```python
from build123d import *

# Parameters (mm, degrees)
SKETCH1_R                  = 45
SKETCH1_R_2                = 5
BOSS_EXTRUDE1_DEPTH        = 8
F_4_3_4_3_DIAMETER_HOLE1_D = 4.3
SKETCH6_R                  = 30.1
SKETCH6_R_2                = 19.9
CUT_EXTRUDE2_DEPTH         = 1.5
SKETCH8_R                  = 24
SKETCH8_R_2                = 12.5
CUT_EXTRUDE3_DEPTH         = 3
SKETCH9_R                  = 24
SKETCH9_R_2                = 14.5
CUT_EXTRUDE4_DEPTH         = 0.6
SKETCH10_R                 = 12.5
SKETCH10_R_2               = 2.15
BOSS_EXTRUDE2_DEPTH        = 14.5
CHAMFER1_SIZE              = 1
FILLET1_R                  = 1


with BuildPart() as part:
    # Sketch1 → Boss-Extrude1 (new body)
    with BuildSketch(Plane(origin=(0, 0, 0), x_dir=(1, 0, 0), z_dir=(0, 1, 0))):
        with Locations(Location((0, 0, 0), (0, 0, 270))):
            Circle(SKETCH1_R)
        with Locations(Location((0, 36.5, 0), (0, 0, 270))):
            Circle(SKETCH1_R_2, mode=Mode.SUBTRACT)
        with Locations(Location((34.713562845, 11.279120295, 0), (0, 0, 270))):
            Circle(SKETCH1_R_2, mode=Mode.SUBTRACT)
        with Locations(Location((21.454161709, -29.529120295, 0), (0, 0, 270))):
            Circle(SKETCH1_R_2, mode=Mode.SUBTRACT)
        with Locations(Location((-21.454161709, -29.529120295, 0), (0, 0, 270))):
            Circle(SKETCH1_R_2, mode=Mode.SUBTRACT)
        with Locations(Location((-34.713562845, 11.279120295, 0), (0, 0, 270))):
            Circle(SKETCH1_R_2, mode=Mode.SUBTRACT)
    extrude(amount=BOSS_EXTRUDE1_DEPTH)

    # Ø4.3 (4.3) Diameter Hole1 (through all)
    with Locations(Plane(origin=(0, 8, 0), x_dir=(1, 0, 0), z_dir=(0, 1, 0))):
        with Locations((-7.60845213, -2.472135955), (-4.702282018, 6.472135955), (4.702282018, 6.472135955), (7.60845213, -2.472135955), (0, -8)):
            Hole(F_4_3_4_3_DIAMETER_HOLE1_D / 2)

    # Sketch6 → Cut-Extrude2 (cut)
    with BuildSketch(Plane.XZ):
        with Locations(Location((0, 0, 0), (0, 0, 270))):
            Circle(SKETCH6_R)
        with Locations(Location((0, 0, 0), (0, 0, 270))):
            Circle(SKETCH6_R_2, mode=Mode.SUBTRACT)
    extrude(amount=-CUT_EXTRUDE2_DEPTH, mode=Mode.SUBTRACT)

    # Sketch8 → Cut-Extrude3 (cut)
    with BuildSketch(Plane(origin=(0, 8, 0), x_dir=(1, 0, 0), z_dir=(0, 1, 0))):
        with Locations(Location((0, 0, 0), (0, 0, 270))):
            Circle(SKETCH8_R)
        with Locations(Location((0, 0, 0), (0, 0, 270))):
            Circle(SKETCH8_R_2, mode=Mode.SUBTRACT)
    extrude(amount=-CUT_EXTRUDE3_DEPTH, mode=Mode.SUBTRACT)

    # Sketch9 → Cut-Extrude4 (cut)
    with BuildSketch(Plane(origin=(0, 5, 0), x_dir=(1, 0, 0), z_dir=(0, 1, 0))):
        with Locations(Location((0, 0, 0), (0, 0, 270))):
            Circle(SKETCH9_R)
        with Locations(Location((0, 0, 0), (0, 0, 270))):
            Circle(SKETCH9_R_2, mode=Mode.SUBTRACT)
    extrude(amount=-CUT_EXTRUDE4_DEPTH, mode=Mode.SUBTRACT)

    # Sketch10 → Boss-Extrude2 (add)
    with BuildSketch(Plane.XZ.offset(-8)):
        with Locations(Location((0, 0, 0), (0, 0, 90))):
            Circle(SKETCH10_R)
        with Locations(Location((7.60845213, 2.472135955, 0), (0, 0, 90))):
            Circle(SKETCH10_R_2, mode=Mode.SUBTRACT)
        with Locations(Location((4.702282018, -6.472135955, 0), (0, 0, 90))):
            Circle(SKETCH10_R_2, mode=Mode.SUBTRACT)
        with Locations(Location((-4.702282018, -6.472135955, 0), (0, 0, 90))):
            Circle(SKETCH10_R_2, mode=Mode.SUBTRACT)
        with Locations(Location((-7.60845213, 2.472135955, 0), (0, 0, 90))):
            Circle(SKETCH10_R_2, mode=Mode.SUBTRACT)
        with Locations(Location((0, 8, 0), (0, 0, 90))):
            Circle(SKETCH10_R_2, mode=Mode.SUBTRACT)
    extrude(amount=-BOSS_EXTRUDE2_DEPTH)

    # Chamfer1
    chamfer1_edges = [part.edges().sort_by_distance(p)[0] for p in [
        (0, 22.5, -12.5),
    ]]
    chamfer(chamfer1_edges, length=CHAMFER1_SIZE)

    # Sketch11 → Cut-Revolve1 (revolve, cut)
    with BuildSketch(Plane.XY, mode=Mode.PRIVATE) as cut_revolve1_sk:
        Polygon((12.5, 5), (12.5, 7), (10.5, 5), align=None)
    revolve(cut_revolve1_sk.sketch.rotate(Axis((0, 1.5, 0), (0, -1, 0)), 90), axis=Axis((0, 1.5, 0), (0, -1, 0)), mode=Mode.SUBTRACT)

    # Fillet1
    fillet1_edges = [part.edges().sort_by_distance(p)[0] for p in [
        (0, 5, -10.5),
    ]]
    fillet(fillet1_edges, radius=FILLET1_R)


solid = part.part
```
Check sheet for the modelled part. Datum: model origin and axes. Units: mm. A direction names the side the tool comes from. Give positions to 0.01 mm unless a question says otherwise; leave off trailing zeros. Order: outer loops, then holes, each group sorted by start corner. A loop starts at its lowest first (then second) coordinate and runs counter-clockwise, first axis right, second up. Notation, with made-up numbers: (-33, -10.75) -> (-27, -10.75) arc R20 ccw to (-27, 23.25) -> close; hole circle Ø3 at (28, 19). An arc over 180 degrees is marked (long way). Use CSV: the item, a comma, the result in double quotes. Start each with the question number.
1) Material ranges on line 1 (X direction, y = 7.5, z = -4); line 2 (Z direction, x = -12, y = 4.5); line 3 (X direction, y = 2, z = 34), recorded low to high. Write a range as from..to.
2) Sectioned sample at B-B, the plane x = -38. Record the boundary of the cut face in (y, z).
3) Set-up check for faces 1 (the face through (-29.384, 0.74, 6.525)), 2 (the face through (9, 5, 10)), 3 (the face through (-0.8, 11.092, 9.996)): record each of +Z, -Z, +X, -X, +Y, -Y from which the full face is reachable in a straight line by a thin tool's end or side.
4) Sectioned sample at A-A, the plane z = -36.5. Record the boundary of the cut face in (x, y).
5) Go/stop test with flat-tipped pins: P1, Ø16, axis at x = -21.45, z = 29.53, coming from the +Y side; P2, Ø6, axis at x = 15, z = -18.5, coming from the -Y side; P3, Ø8, axis at x = 3, y = 11, coming from the +Z side. Record where each tip stops, or that it passes through.
6) Sectioned sample at C-C, the plane y = 17.25. Record the boundary of the cut face in (x, z), plus the area to 3 significant figures.
7) Sectioned sample at D-D, the plane z = -26. Record the boundary of the cut face in (x, y).
Recorded:
1,line 1,"-44.82..-23.66, -11.84..11.84, 23.66..44.82"
1,line 2,"-43.37..-20.78, -8.14..8.14, 20.78..43.37"
1,line 3,"-29.48..-23.69, -19.22..19.22, 23.69..29.48"
2,outline,"(0, -24.1) -> (8, -24.1) -> (8, -15.05) -> (0, -15.05) -> close; (0, -7.51) -> (8, -7.51) -> (8, 24.1) -> (0, 24.1) -> close"
3,face 1,"-Y"
3,face 2,"+Y"
3,face 3,"+Y, -Y"
4,outline,"(-26.32, 0) -> (-5, 0) -> (-5, 8) -> (-26.32, 8) -> close; (5, 0) -> (26.32, 0) -> (26.32, 8) -> (5, 8) -> close"
5,P1,"y = 8"
5,P2,"y = 1.5"
5,P3,"z = 45"
6,outline,"circle Ø25 at (0, 0); hole circle Ø4.3 at (-7.61, 2.47); hole circle Ø4.3 at (-4.7, -6.47); hole circle Ø4.3 at (0, 8); hole circle Ø4.3 at (4.7, -6.47); hole circle Ø4.3 at (7.61, 2.47)"
6,area,"418 mm2"
7,outline,"(-36.73, 0) -> (-15.17, 0) -> (-15.17, 1.5) -> (15.17, 1.5) -> (15.17, 0) -> (36.73, 0) -> (36.73, 8) -> (-36.73, 8) -> close"
